Check sheet for the modelled part. Datum: model origin and axes. Units: mm. Face numbers are marked on the shaded views. A direction names the side the tool comes from. Coordinates: 2 decimals unless noted, no trailing zeros. Write each loop counter-clockwise with the first axis right and the second up, starting at its lowest first coordinate (ties: lowest second). Pieces come first, ordered by that corner, then holes. Notation, with made-up numbers: (15, -10.75) -> (41, -10.75) arc R9 ccw to (41, -4.75) -> close; hole circle Ø11 at (38.25, -39). An arc over 180 degrees is marked (long way). Put each result on its own line as item: value.
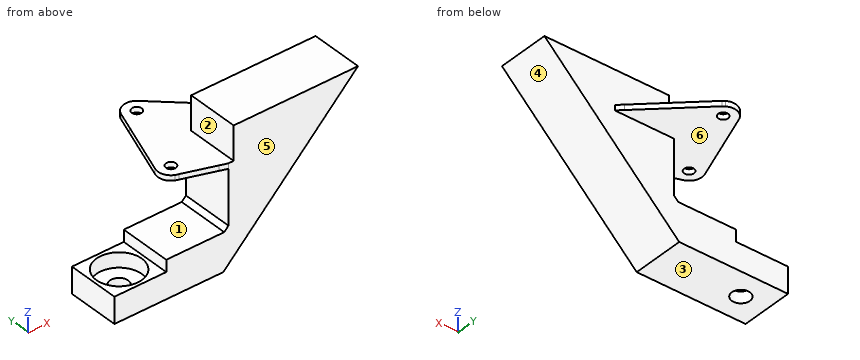
```python
from build123d import *

# Parameters (mm, degrees)
BOSS_EXTRUDE1_DEPTH = 25.4
SKETCH2_R           = 11.1125
CUT_EXTRUDE1_DEPTH  = 7.1628
CUT_EXTRUDE2_REACH  = 123.946
SKETCH2_3_R         = 4.445
BOSS_EXTRUDE2_DEPTH = 68.58
CUT_EXTRUDE3_REACH  = 138.151
SKETCH4_R           = 2.413
CUT_EXTRUDE4_REACH  = 138.151
CUT_EXTRUDE5_START  = 16.51
CUT_EXTRUDE5_DEPTH  = 16.51
CUT_EXTRUDE7_REACH  = 131.829
CUT_EXTRUDE8_REACH  = 155.739
CUT_EXTRUDE10_REACH = 131.829
BOSS_EXTRUDE3_DEPTH = 2.54


with BuildPart() as part:
    # Sketch1 → Boss-Extrude1 (new body)
    with BuildSketch(Plane(origin=(0, 0, 0), x_dir=(1, 0, 0), z_dir=(0, 1, 0))):
        Polygon((35.379487758, -53.34), (22.679487758, -40.64), (-12.7, -40.64), (-12.7, -53.34), (12.7, -53.34), align=None)
        Polygon((90.17, -90.17), (40.64, -40.64), (22.679487758, -40.64), (35.379487758, -53.34), (41.094487758, -59.055), (43.18, -61.140512242), (72.209487758, -90.17), align=None)
        Polygon((41.094487758, -59.055), (35.379487758, -53.34), (12.7, -53.34), (12.7, -59.055), align=None)
        Polygon((45.72, -90.17), (72.209487758, -90.17), (43.18, -61.140512242), (43.18, -87.63), (16.51, -87.63), (16.51, -90.17), align=None)
        Polygon((88.719487758, -106.68), (72.209487758, -90.17), (45.72, -90.17), (45.72, -106.68), align=None)
        Polygon((106.68, -106.68), (90.17, -90.17), (72.209487758, -90.17), (88.719487758, -106.68), align=None)
    extrude(amount=BOSS_EXTRUDE1_DEPTH)

    # Sketch2 → Cut-Extrude1 (cut)
    with BuildSketch(Plane.XY.offset(53.34)):
        with Locations((0, 12.7)):
            Circle(SKETCH2_R)
    extrude(amount=-CUT_EXTRUDE1_DEPTH, mode=Mode.SUBTRACT)

    # Sketch2<3> → Cut-Extrude2 (cut, up to next)
    with BuildSketch(Plane.XY.offset(53.34), mode=Mode.PRIVATE) as cut_extrude2_sk1:
        with Locations((0, 12.7)):
            Circle(SKETCH2_3_R)
    cut_extrude2_tool1 = extrude(cut_extrude2_sk1.sketch, amount=-CUT_EXTRUDE2_REACH, mode=Mode.PRIVATE) & part.part
    add(cut_extrude2_tool1.solids().sort_by_distance((0, 12.7, 53.34))[0], mode=Mode.SUBTRACT)

    # Sketch1<3> → Boss-Extrude2 (add)
    with BuildSketch(Plane(origin=(0, 0, 0), x_dir=(1, 0, 0), z_dir=(0, 1, 0))):
        Polygon((88.719487758, -106.68), (72.209487758, -90.17), (45.72, -90.17), (45.72, -106.68), align=None)
        Polygon((45.72, -90.17), (72.209487758, -90.17), (43.18, -61.140512242), (43.18, -87.63), (16.51, -87.63), (16.51, -90.17), align=None)
    extrude(amount=BOSS_EXTRUDE2_DEPTH)

    # Sketch4 → Cut-Extrude3 (cut, up to next)
    with BuildSketch(Plane.XY.offset(90.17), mode=Mode.PRIVATE) as cut_extrude3_sk1:
        with Locations((38.1, 48.621024484)):
            Circle(SKETCH4_R)
    cut_extrude3_tool1 = extrude(cut_extrude3_sk1.sketch, amount=-CUT_EXTRUDE3_REACH, mode=Mode.PRIVATE) & part.part
    # Sketch4 → Cut-Extrude3 (cut, up to next)
    with BuildSketch(Plane.XY.offset(90.17), mode=Mode.PRIVATE) as cut_extrude3_sk2:
        with Locations((25.4, 12.7)):
            Circle(SKETCH4_R)
    cut_extrude3_tool2 = extrude(cut_extrude3_sk2.sketch, amount=-CUT_EXTRUDE3_REACH, mode=Mode.PRIVATE) & part.part
    add(cut_extrude3_tool1.solids().sort_by_distance((38.1, 48.621024, 90.17))[0], mode=Mode.SUBTRACT)
    add(cut_extrude3_tool2.solids().sort_by_distance((25.4, 12.7, 90.17))[0], mode=Mode.SUBTRACT)

    # Sketch4<4> → Cut-Extrude4 (cut, up to next)
    with BuildSketch(Plane.XY.offset(90.17), mode=Mode.PRIVATE) as cut_extrude4_sk1:
        with BuildLine():
            ThreePointArc((16.51, 50.529162362), (23.165769401, 46.860982905), (29.036193408, 42.034708067))
            Line((29.036193408, 42.034708067), (32.113162586, 50.737691151))
            ThreePointArc((32.113162586, 50.737691151), (35.962630111, 54.600501883), (41.388506693, 54.053171733))
            Line((41.388506693, 54.053171733), (88.719487758, 25.4))
            Line((88.719487758, 25.4), (88.719487758, 68.58))
            Line((88.719487758, 68.58), (16.51, 68.58))
            Line((16.51, 68.58), (16.51, 50.529162362))
        make_face()
    cut_extrude4_tool1 = extrude(cut_extrude4_sk1.sketch, amount=-CUT_EXTRUDE4_REACH, mode=Mode.PRIVATE) & part.part
    # Sketch4<4> → Cut-Extrude4 (cut, up to next)
    with BuildSketch(Plane.XY.offset(90.17), mode=Mode.PRIVATE) as cut_extrude4_sk2:
        with BuildLine():
            ThreePointArc((24.141722061, 6.475914796), (23.355096734, 6.688272242), (22.602138971, 6.999607587))
            ThreePointArc((22.602138971, 6.999607587), (19.520430726, 10.301424349), (19.413162586, 14.816666667))
            Line((19.413162586, 14.816666667), (29.036193408, 42.034708067))
            ThreePointArc((29.036193408, 42.034708067), (23.165769401, 46.860982905), (16.51, 50.529162362))
            Line((16.51, 50.529162362), (16.51, 0))
            Line((16.51, 0), (39.272581084, 0))
            ThreePointArc((39.272581084, 0), (39.461690116, 0.600386859), (39.64162121, 1.203587826))
            Line((39.64162121, 1.203587826), (24.141722061, 6.475914796))
        make_face()
    cut_extrude4_tool2 = extrude(cut_extrude4_sk2.sketch, amount=-CUT_EXTRUDE4_REACH, mode=Mode.PRIVATE) & part.part
    add(cut_extrude4_tool1.solids().sort_by_distance((58.41037, 54.420035, 90.17))[0], mode=Mode.SUBTRACT)
    add(cut_extrude4_tool2.solids().sort_by_distance((21.980861, 24.151697, 90.17))[0], mode=Mode.SUBTRACT)

    # Sketch4<7> → Cut-Extrude5 (cut)
    with BuildSketch(Plane.XY.offset(90.17).offset(CUT_EXTRUDE5_START)):
        with BuildLine():
            ThreePointArc((16.51, 50.529162362), (23.165769401, 46.860982905), (29.036193408, 42.034708067))
            Line((29.036193408, 42.034708067), (32.113162586, 50.737691151))
            ThreePointArc((32.113162586, 50.737691151), (35.962630111, 54.600501883), (41.388506693, 54.053171733))
            Line((41.388506693, 54.053171733), (88.719487758, 25.4))
            Line((88.719487758, 25.4), (88.719487758, 68.58))
            Line((88.719487758, 68.58), (16.51, 68.58))
            Line((16.51, 68.58), (16.51, 50.529162362))
        make_face()
        with BuildLine():
            ThreePointArc((24.141722061, 6.475914796), (23.355096734, 6.688272242), (22.602138971, 6.999607587))
            ThreePointArc((22.602138971, 6.999607587), (19.520430726, 10.301424349), (19.413162586, 14.816666667))
            Line((19.413162586, 14.816666667), (29.036193408, 42.034708067))
            ThreePointArc((29.036193408, 42.034708067), (23.165769401, 46.860982905), (16.51, 50.529162362))
            Line((16.51, 50.529162362), (16.51, 0))
            Line((16.51, 0), (39.272581084, 0))
            ThreePointArc((39.272581084, 0), (39.461690116, 0.600386859), (39.64162121, 1.203587826))
            Line((39.64162121, 1.203587826), (24.141722061, 6.475914796))
        make_face()
        with BuildLine():
            Line((43.18, 0), (39.64162121, 1.203587826))
            ThreePointArc((39.64162121, 1.203587826), (39.461690116, 0.600386859), (39.272581084, 0))
            Line((39.272581084, 0), (43.18, 0))
        make_face()
    extrude(amount=-CUT_EXTRUDE5_DEPTH, mode=Mode.SUBTRACT)

    # Sketch4<10> → Cut-Extrude7 (cut, up to next)
    with BuildSketch(Plane.XY.offset(90.17), mode=Mode.PRIVATE) as cut_extrude7_sk1:
        with BuildLine():
            Line((43.18, 0), (39.64162121, 1.203587826))
            ThreePointArc((39.64162121, 1.203587826), (39.461690116, 0.600386859), (39.272581084, 0))
            Line((39.272581084, 0), (43.18, 0))
        make_face()
    cut_extrude7_tool1 = extrude(cut_extrude7_sk1.sketch, amount=-CUT_EXTRUDE7_REACH, mode=Mode.PRIVATE) & part.part
    add(cut_extrude7_tool1.solids().sort_by_distance((40.700194, 0.400853, 90.17))[0], mode=Mode.SUBTRACT)

    # Sketch7 → Cut-Extrude8 (cut, up to next)
    with BuildSketch(Plane(origin=(0, 25.4, 0), x_dir=(1, 0, 0), z_dir=(0, 1, 0)), mode=Mode.PRIVATE) as cut_extrude8_sk1:
        Polygon((43.18, -61.140512242), (43.18, -87.63), (69.669487758, -87.63), align=None)
    cut_extrude8_tool1 = extrude(cut_extrude8_sk1.sketch, amount=CUT_EXTRUDE8_REACH, mode=Mode.PRIVATE) & part.part
    # Sketch7 → Cut-Extrude8 (cut, up to next)
    with BuildSketch(Plane(origin=(0, 25.4, 0), x_dir=(1, 0, 0), z_dir=(0, 1, 0)), mode=Mode.PRIVATE) as cut_extrude8_sk2:
        Polygon((45.72, -90.17), (72.209487758, -90.17), (88.719487758, -106.68), (45.72, -106.68), align=None)
    cut_extrude8_tool2 = extrude(cut_extrude8_sk2.sketch, amount=CUT_EXTRUDE8_REACH, mode=Mode.PRIVATE) & part.part
    add(cut_extrude8_tool1.solids().sort_by_distance((52.009829, 25.4, 78.800171))[0], mode=Mode.SUBTRACT)
    add(cut_extrude8_tool2.solids().sort_by_distance((63.41913, 25.4, 99.078773))[0], mode=Mode.SUBTRACT)

    # Sketch8 → Cut-Extrude10 (cut, up to next)
    with BuildSketch(Plane.XY.offset(90.17), mode=Mode.PRIVATE) as cut_extrude10_sk1:
        with BuildLine():
            Line((69.540863311, 27.897131539), (72.209487758, 25.4))
            Line((72.209487758, 25.4), (72.209487758, 35.394803713))
            Line((72.209487758, 35.394803713), (41.388506693, 54.053171733))
            ThreePointArc((41.388506693, 54.053171733), (41.934277279, 53.682725557), (42.438674479, 53.257661602))
            Line((42.438674479, 53.257661602), (69.540863311, 27.897131539))
        make_face()
    cut_extrude10_tool1 = extrude(cut_extrude10_sk1.sketch, amount=-CUT_EXTRUDE10_REACH, mode=Mode.PRIVATE) & part.part
    add(cut_extrude10_tool1.solids().sort_by_distance((62.122661, 38.169884, 90.17))[0], mode=Mode.SUBTRACT)

    # Sketch8<3> → Boss-Extrude3 (add)
    with BuildSketch(Plane.XY.offset(90.17)):
        Polygon((69.540863311, 25.4), (72.209487758, 25.4), (69.540863311, 27.897131539), align=None)
    extrude(amount=-BOSS_EXTRUDE3_DEPTH)


solid = part.part
```
Q1. Mould release check, pull along Z, two halves, no side actions. Record for the marked faces 4, 5 and 6: released by +Z, released by -Z, zero draft, split by the parting line, or undercut.
Recorded:
face 4: released by -Z
face 5: zero draft
face 6: undercut
Q2. Cross-section at A-A (y = 12.7). State how many separate pieces and enclosed holes the cut face has, plus the area to 3 significant figures.
Recorded:
separate pieces: 3
enclosed holes: 0
area: 2,700 mm2
Q3. Cross-section at C-C (x = 38.1). Record the cut outline in (y, z) (3 decimals).
Recorded:
outline: (0, 40.64) -> (25.4, 40.64) -> (25.4, 59.055) -> (0, 59.055) -> close; (1.728, 87.63) -> (46.208, 87.63) -> (46.208, 90.17) -> (1.728, 90.17) -> close; (51.034, 87.63) -> (54.971, 87.63) -> (54.971, 90.17) -> (51.034, 90.17) -> close
Q4. Depth check by flat-ended pin: P1, Ø20.5, axis at x = 26.5, y = 9, coming from the +Z side; P2, Ø1.5, axis at x = 87, y = 10, coming from the -Z side; P3, Ø11, axis at x = -5, y = 8, coming from the +Z side; P4, Ø4, axis at x = 38.1, y = 48.62, coming from the +Z side. Enter the tip coordinate at first touch or a pass-through.
Recorded:
P1: stops at z = 90.17
P2: stops at z = 86.25
P3: stops at z = 53.34
P4: passes through
Q5. Cross-section at B-B (x = 1.5). Record the cut outline in (y, z).
Recorded:
outline: (0, 40.64) -> (8.52, 40.64) -> (8.52, 46.18) -> (1.69, 46.18) -> (1.69, 53.34) -> (0, 53.34) -> close; (16.88, 40.64) -> (25.4, 40.64) -> (25.4, 53.34) -> (23.71, 53.34) -> (23.71, 46.18) -> (16.88, 46.18) -> close
Q6. Cross-section at D-D (z = 71). Record the cut outline in (x, y), plus the area to 3 significant figures.
Recorded:
outline: (43.18, 0) -> (71, 0) -> (71, 25.4) -> (43.18, 25.4) -> close
area: 707 mm2
Q7. Material ranges on line 1 along Z through (x, y) = (36.5, 20.5) (3 decimals); line 2 along Y through (x, z) = (50.5, 78.5); line 3 along Z through (x, y) = (10, 4.5), recorded low to high.
Recorded:
line 1: z = 40.64 to 59.055, 87.63 to 90.17
line 2: y = 0 to 25.4
line 3: z = 40.64 to 53.34
Q8. Tool access check on the marked faces 1, 2 and 3. Record the directions out of +Z, -Z, +X, -X, +Y, -Y that give a thin tool (end or side, any length) a straight path to the whole face; none if there is none.
Recorded:
face 1: -X, +Y, -Y
face 2: +Z, -X, +Y, -Y
face 3: -Z, +X, -X, +Y, -Y
